Check sheet for the modelled part. Datum: model origin and axes. Units: mm. A direction names the side the tool comes from. Coordinates: 2 decimals unless noted, no trailing zeros. Loops run counter-clockwise (first coordinate to the right, second up) from the corner with the lowest first, then second, coordinate; pieces in that order, holes last.
from build123d import *

# Parameters (mm, degrees)
SKETCH_W         = 91
SKETCH_H         = 8.5
PAD_DEPTH        = 19
FILLET_R         = 7
SKETCH052_R      = 1.6
POCKET_DEPTH     = 8
HOLE_D           = 3.3
HOLE_DEPTH       = 25
HOLE_CSINK_D     = 6.1
HOLE_CSINK_ANGLE = 90


with BuildPart() as part:
    # Sketch → Pad (new body)
    with BuildSketch(Plane.XY):
        with Locations((45.5, 4.25)):
            Rectangle(SKETCH_W, SKETCH_H)
    extrude(amount=PAD_DEPTH)

    # Fillet
    fillet_edges = [part.edges().sort_by_distance(p)[0] for p in [
        (91, 8.5, 9.5),
        (0, 8.5, 9.5),
    ]]
    fillet(fillet_edges, radius=FILLET_R)

    # Sketch052 (on Face5 of Fillet) → Pocket (cut)
    with BuildSketch(Plane.XY.offset(19)):
        with Locations((4.749754, 4.25)):
            Circle(SKETCH052_R)
        with Locations((86.299538, 4.25)):
            Circle(SKETCH052_R)
        with Locations((43.855799, 4.26)):
            Circle(SKETCH052_R)
    extrude(amount=-POCKET_DEPTH, mode=Mode.SUBTRACT)

    # Hole
    with Locations(Plane.XZ):
        with Locations((22.75, 10), (68.249998, 10)):
            CounterSinkHole(HOLE_D / 2, HOLE_CSINK_D / 2, depth=HOLE_DEPTH, counter_sink_angle=HOLE_CSINK_ANGLE)


solid = part.part
(1) Draft check along Z on faces 3 (the face through (2, 6.4, 9.6)), 4 (the face through (45, 2, 19)), 5 (the face through (66.726, 5, 9.368)). Enter one of: pulls with the +Z half, pulls with the -Z half, needs draft (parallel to the pull), parting line crosses it, or undercut.
(2) Section check A-A, the plane z = 17. Enter the section's corners in (x, y).
(3) Set-up check for faces 1 (the face through (45, 4, 0)), 2 (the face through (5, 4, 11)): record each of +Z, -Z, +X, -X, +Y, -Y from which the full face is reachable in a straight line by a thin tool's end or side.
(4) Section check D-D, the plane z = 2.5. Enter the section's corners in (x, y), plus the area to 3 significant figures.
(5) Section check C-C, the plane y = 7.25. Enter the section's corners in (x, z), plus the area to 3 significant figures.
(6) Gauge pin test, flat ends, axial feed: P1, Ø5.5, axis at x = 22.75, z = 10, coming from the -Y side; P2, Ø3, axis at y = 5.5, z = 3.5, coming from the -X side; P3, Ø5, axis at y = 5, z = 4, coming from the -X side. Record the tip position at first contact, or that the pin passes through.
(7) Scan lines: line 1 along X through (y, z) = (1.25, 10); line 2 along X through (y, z) = (4.75, 16.75); line 3 along X through (y, z) = (0.5, 9). Record each from-to range of solid material in increasing order.
(8) Section check B-B, the plane z = 10. Enter the section's corners in (x, y), plus the area to 3 significant figures.
Determined:
1. face 3: needs draft
1. face 4: pulls with the +Z half
1. face 5: undercut
2. outline: (0, 0) - (91, 0) - (91, 1.5) arc R7 ccw to (84, 8.5) - (7, 8.5) arc R7 ccw to (0, 1.5) - close; hole circle Ø3.2 at (4.75, 4.25); hole circle Ø3.2 at (43.86, 4.26); hole circle Ø3.2 at (86.3, 4.25)
3. face 1: -Z, +X, -X, +Y, -Y
3. face 2: +Z
4. outline: (0, 0) - (91, 0) - (91, 1.5) arc R7 ccw to (84, 8.5) - (7, 8.5) arc R7 ccw to (0, 1.5) - close
4. area: 752 mm2
5. outline: (3.01, 0) - (87.99, 0) - (87.99, 19) - (3.01, 19) - close; hole circle Ø3.3 at (22.75, 10); hole circle Ø3.3 at (68.25, 10)
5. area: 1,600 mm2
6. P1: stops at y = 0.3
6. P2: stops at x = 0.46
6. P3: stops at x = 0.07
7. line 1: x = 0 to 20.95, 24.55 to 66.45, 70.05 to 91
7. line 2: x = 0.8 to 3.23, 6.27 to 42.33, 45.38 to 84.78, 87.82 to 90.2
7. line 3: x = 0 to 20.4, 25.1 to 65.9, 70.6 to 91
8. outline: (0, 0) - (19.7, 0) - (21.1, 1.4) - (21.1, 8.5) - (7, 8.5) arc R7 ccw to (0, 1.5) - close; (24.4, 1.4) - (25.8, 0) - (65.2, 0) - (66.6, 1.4) - (66.6, 8.5) - (24.4, 8.5) - close; (69.9, 1.4) - (71.3, 0) - (91, 0) - (91, 1.5) arc R7 ccw to (84, 8.5) - (69.9, 8.5) - close
8. area: 692 mm2
